```python
from build123d import *

# Parameters (mm, degrees)
F1_W      = 86
F1_H      = 86
F1_R      = 2.75
F2_DEPTH  = 8.5
F3_R      = 36.5
F4_DEPTH  = 1.5
F5_R      = 7
F6_DEPTH  = 37
F8_DEPTH  = 113
F9_R      = 5.5
F10_R     = 3.175
F11_DEPTH = 13.5


with BuildPart() as f2:
    # F1 (on Front) → F2 (new body)
    with BuildSketch(Plane.XZ):
        Rectangle(F1_W, F1_H)
        with Locations((-34.8, -34.8)):
            Circle(F1_R, mode=Mode.SUBTRACT)
        with Locations((34.8, -34.8)):
            Circle(F1_R, mode=Mode.SUBTRACT)
        with Locations((-34.8, 34.8)):
            Circle(F1_R, mode=Mode.SUBTRACT)
        with Locations((34.8, 34.8)):
            Circle(F1_R, mode=Mode.SUBTRACT)
    extrude(amount=-F2_DEPTH)

    # F3 (on Front) → F4 (join)
    with BuildSketch(Plane.XZ):
        Circle(F3_R)
    extrude(amount=F4_DEPTH)

    # F5 (on Front) → F6 (join)
    with BuildSketch(Plane.XZ):
        Circle(F5_R)
    extrude(amount=F6_DEPTH)

    # F7 (on Front) → F8 (join)
    with BuildSketch(Plane.XZ):
        with BuildLine():
            ThreePointArc((34.8, 29.3), (30.9109127035, 30.9109127035), (29.3, 34.8))
            Line((29.3, 34.8), (29.3, 43))
            Line((29.3, 43), (-29.3, 43))
            Line((-29.3, 43), (-29.3, 34.8))
            ThreePointArc((-29.3, 34.8), (-30.9109127035, 30.9109127035), (-34.8, 29.3))
            Line((-34.8, 29.3), (-43, 29.3))
            Line((-43, 29.3), (-43, -29.3))
            Line((-43, -29.3), (-34.8, -29.3))
            ThreePointArc((-34.8, -29.3), (-30.9109127035, -30.9109127035), (-29.3, -34.8))
            Line((-29.3, -34.8), (-29.3, -43))
            Line((-29.3, -43), (29.3, -43))
            Line((29.3, -43), (29.3, -34.8))
            ThreePointArc((29.3, -34.8), (30.9109127035, -30.9109127035), (34.8, -29.3))
            Line((34.8, -29.3), (43, -29.3))
            Line((43, -29.3), (43, 29.3))
            Line((43, 29.3), (34.8, 29.3))
        make_face()
    extrude(amount=-F8_DEPTH)

    # F9
    f9_edges = [f2.edges().sort_by_distance(p)[0] for p in [
        (29.3, 60.75, 43),
        (43, 60.75, 29.3),
        (43, 4.25, 43),
        (-29.3, 60.75, 43),
        (-43, 60.75, 29.3),
        (-43, 4.25, 43),
        (43, 60.75, -29.3),
        (29.3, 60.75, -43),
        (-43, 4.25, -43),
        (-29.3, 60.75, -43),
        (-43, 60.75, -29.3),
        (43, 4.25, -43),
    ]]
    fillet(f9_edges, radius=F9_R)

    # F10 (on face) → F11 (join)
    with BuildSketch(Plane(origin=(0, 113, 0), x_dir=(-1, 0, 0), z_dir=(0, 1, 0))):
        Circle(F10_R)
    extrude(amount=F11_DEPTH)


solid = f2.part
```
For this review, take the finished solid that the model builds, in its own axes (mm). A direction names the side the tool comes from. Give positions to 0.01 mm unless a question says otherwise; leave off trailing zeros. Write each loop counter-clockwise with the first axis right and the second up, starting at its lowest first coordinate (ties: lowest second). Pieces come first, ordered by that corner, then holes. Notation, with made-up numbers: M -2,-33 L 7,-33 A16 ccw 7,-28 Z; hole C -19.75,4 d2. An arc over 180 degrees is marked long. One line per item, written item: value.
1) For faces 1 (the cylindrical face through (27.73, 61.48, 41.35)), 2 (the flat face through (43, 56, -1)), 3 (the cylindrical face through (-41.35, 61.48, -27.73)), 4 (the cylindrical face through (-7.912, -0.74, -35.632)), 5 (the flat face through (-36, 8.5, 38)), list the 3-axis set-ups (+Z, -Z, +X, -X, +Y, -Y) from which the entire face can be reached by the end or side of a thin tool; tool diameter is ignored.
Results are:
face 1: +Z, +X, +Y
face 2: +Z, -Z, +X, +Y, -Y
face 3: -Z, -X, +Y
face 4: -Y
face 5: +Z, -X, +Y
2) Take a section at B-B, the plane x = 0. Write out the cut boundary in (y, z) (3 decimals).
Results are:
outline: M -37,-7 L -1.5,-7 L -1.5,-36.5 L 0,-36.5 L 0,-43 L 113,-43 L 113,-3.175 L 126.5,-3.175 L 126.5,3.175 L 113,3.175 L 113,43 L 0,43 L 0,36.5 L -1.5,36.5 L -1.5,7 L -37,7 Z
3) Take a section at A-A, the plane z = 0. Write out the cut boundary in (x, y) (3 decimals), then the cut area to 3 significant figures.
Results are:
outline: M -43,0 L -36.5,0 L -36.5,-1.5 L -7,-1.5 L -7,-37 L 7,-37 L 7,-1.5 L 36.5,-1.5 L 36.5,0 L 43,0 L 43,113 L 3.175,113 L 3.175,126.5 L -3.175,126.5 L -3.175,113 L -43,113 Z
area: 10,400 mm²
4) For P1, Ø1.4, axis at y = 73, z = -36.5, coming from the -X side; P2, Ø5, axis at x = 31, y = 53, coming from the +Z side; P3, Ø21, axis at x = -31, z = 34.5, coming from the +Y side; P4, Ø4.5, axis at x = 34.8, z = -34.8, coming from the +Y side, all flat-tipped, find the tip position at first contact; note any pin that passes through.
Results are:
P1: stops at x = -29.3
P2: stops at z = 40.36
P3: stops at y = 113
P4: passes through
5) Take a section at D-D, the plane z = -13.5. Write out the cut boundary in (x, y), then the cut area to 3 significant figures.
Results are:
outline: M -43,0 L -33.91,0 L -33.91,-1.5 L 33.91,-1.5 L 33.91,0 L 43,0 L 43,113 L -43,113 Z
area: 9,820 mm²
6) The part is to be moulded in two halves that separate along X. For faces 6 (the cylindrical face through (-30.87, 60.02, 30.95)), 7 (the cylindrical face through (41.43, 4.31, -41.35)), 8 (the cylindrical face through (-35.396, 4.19, -37.485)), 9 (the flat face through (38, 8.5, -35)), say which applies: +X half, -X half, draft (parallel to the pull), parting line (faces both ways), or undercut.
Results are:
face 6: -X half
face 7: +X half
face 8: undercut
face 9: draft
7) Take a section at C-C, the plane y = 56. Write out the cut boundary in (x, z).
Results are:
outline: M -43,-23.8 A5.5 ccw -37.5,-29.3 L -34.8,-29.3 A5.5 cw -29.3,-34.8 L -29.3,-37.5 A5.5 ccw -23.8,-43 L 23.8,-43 A5.5 ccw 29.3,-37.5 L 29.3,-34.8 A5.5 cw 34.8,-29.3 L 37.5,-29.3 A5.5 ccw 43,-23.8 L 43,23.8 A5.5 ccw 37.5,29.3 L 34.8,29.3 A5.5 cw 29.3,34.8 L 29.3,37.5 A5.5 ccw 23.8,43 L -23.8,43 A5.5 ccw -29.3,37.5 L -29.3,34.8 A5.5 cw -34.8,29.3 L -37.5,29.3 A5.5 ccw -43,23.8 Z
8) For line 1 (Z direction, x = 34.8, y = 4.5); line 2 (Z direction, x = 34, y = 6), list the stretches that pass through material, from the lowest coordinate up. Write a range as from..to.
Results are:
line 1: z = -43..-37.55, -32.05..32.05, 37.55..43
line 2: z = -43..-37.43, -32.17..32.17, 37.43..43
